```python
from build123d import *

# Parameters (mm, degrees)
SKETCH1_R          = 2.54
EXTRUDE1_DEPTH     = 20.574
SKETCH2_R          = 19.05
EXTRUDE2_DEPTH     = 1.524
SKETCH3_R          = 3.175
EXTRUDE3_DEPTH     = 20.574
EXTRUDE4_START     = -36.068
EXTRUDE4_DEPTH     = 36.068
FILLET1_R          = 2.54
EXTRUDE5_START     = 14.986
SKETCH5_R          = 3.175
EXTRUDE5_DEPTH     = 14.986
SKETCH6_R          = 1.07823
EXTRUDE6_DEPTH     = 3.81
SKETCH9_W          = 27.159483829
SKETCH9_H          = 18.094101739
CUT_EXTRUDE1_DEPTH = 56.642


with BuildPart() as part:
    # Sketch1 → Extrude1 (new, symmetric)
    with BuildSketch(Plane.XY):
        with BuildLine():
            Line((-23.5712, 28.575), (23.5712, 28.575))
            ThreePointArc((23.5712, 28.575), (27.109420912, 27.109420912), (28.575, 23.5712))
            Line((28.575, 23.5712), (28.575, -23.5712))
            ThreePointArc((28.575, -23.5712), (27.109420912, -27.109420912), (23.5712, -28.575))
            Line((23.5712, -28.575), (-23.5712, -28.575))
            ThreePointArc((-23.5712, -28.575), (-27.109420912, -27.109420912), (-28.575, -23.5712))
            Line((-28.575, -23.5712), (-28.575, 23.5712))
            ThreePointArc((-28.575, 23.5712), (-27.109420912, 27.109420912), (-23.5712, 28.575))
        make_face()
        with Locations((-23.5712, 23.5712)):
            Circle(SKETCH1_R, mode=Mode.SUBTRACT)
        with Locations((23.5712, 23.5712)):
            Circle(SKETCH1_R, mode=Mode.SUBTRACT)
        with Locations((23.5712, -23.5712)):
            Circle(SKETCH1_R, mode=Mode.SUBTRACT)
        with Locations((-23.5712, -23.5712)):
            Circle(SKETCH1_R, mode=Mode.SUBTRACT)
    extrude(amount=EXTRUDE1_DEPTH, both=True)

    # Sketch2 → Extrude2 (add)
    with BuildSketch(Plane.XY.offset(20.574)):
        with Locations(Location((0, 0, 0), (0, 0, 180))):
            Circle(SKETCH2_R)
    extrude(amount=EXTRUDE2_DEPTH)

    # Sketch3 → Extrude3 (add)
    with BuildSketch(Plane.XY.offset(20.574)):
        Circle(SKETCH3_R)
    extrude(amount=EXTRUDE3_DEPTH)

    # Sketch4 → Extrude4 (cut)
    with BuildSketch(Plane(origin=(0, 0, -20.574), x_dir=(-1, 0, 0), z_dir=(0, 0, -1)).offset(EXTRUDE4_START)):
        with BuildLine():
            Line((-23.5712, 18.5674), (-28.575, 18.5674))
            Line((-28.575, 18.5674), (-28.575, 23.5712))
            ThreePointArc((-28.575, 23.5712), (-27.109420912, 27.109420912), (-23.5712, 28.575))
            Line((-23.5712, 28.575), (-18.5674, 28.575))
            Line((-18.5674, 28.575), (-18.5674, 23.5712))
            ThreePointArc((-18.5674, 23.5712), (-20.032979088, 20.032979088), (-23.5712, 18.5674))
        make_face()
        with BuildLine():
            Line((23.5712, 18.5674), (28.575, 18.5674))
            Line((28.575, 18.5674), (28.575, 23.5712))
            ThreePointArc((28.575, 23.5712), (27.109420912, 27.109420912), (23.5712, 28.575))
            Line((23.5712, 28.575), (18.5674, 28.575))
            Line((18.5674, 28.575), (18.5674, 23.5712))
            ThreePointArc((18.5674, 23.5712), (20.032979088, 20.032979088), (23.5712, 18.5674))
        make_face()
        with BuildLine():
            Line((23.5712, -18.5674), (28.575, -18.5674))
            Line((28.575, -18.5674), (28.575, -23.5712))
            ThreePointArc((28.575, -23.5712), (27.109420912, -27.109420912), (23.5712, -28.575))
            Line((23.5712, -28.575), (18.5674, -28.575))
            Line((18.5674, -28.575), (18.5674, -23.5712))
            ThreePointArc((18.5674, -23.5712), (20.032979088, -20.032979088), (23.5712, -18.5674))
        make_face()
        with BuildLine():
            Line((-18.5674, -23.5712), (-18.5674, -28.575))
            Line((-18.5674, -28.575), (-23.5712, -28.575))
            ThreePointArc((-23.5712, -28.575), (-27.109420912, -27.109420912), (-28.575, -23.5712))
            Line((-28.575, -23.5712), (-28.575, -18.5674))
            Line((-28.575, -18.5674), (-23.5712, -18.5674))
            ThreePointArc((-23.5712, -18.5674), (-20.032979088, -20.032979088), (-18.5674, -23.5712))
        make_face()
    extrude(amount=EXTRUDE4_DEPTH, mode=Mode.SUBTRACT)

    # Fillet1
    fillet1_edges = [part.edges().sort_by_distance(p)[0] for p in [
        (28.575, -18.5674, -2.54),
        (18.5674, -28.575, -2.54),
        (18.5674, 28.575, -2.54),
        (28.575, 18.5674, -2.54),
        (-28.575, 18.5674, -2.54),
        (-18.5674, 28.575, -2.54),
        (-18.5674, -28.575, -2.54),
        (-28.575, -18.5674, -2.54),
    ]]
    fillet(fillet1_edges, radius=FILLET1_R)

    # Sketch5 → Extrude5 (add)
    with BuildSketch(Plane(origin=(0, 0, -20.574), x_dir=(-1, 0, 0), z_dir=(0, 0, -1)).offset(EXTRUDE5_START)):
        with Locations(Location((0, 0, 0), (0, 0, 180))):
            Circle(SKETCH5_R)
    extrude(amount=-EXTRUDE5_DEPTH)

    # Sketch6 → Extrude6 (cut)
    with BuildSketch(Plane(origin=(0, 0, -20.574), x_dir=(-1, 0, 0), z_dir=(0, 0, -1))):
        with Locations((-23.0124, 0)):
            Circle(SKETCH6_R)
        with Locations((23.0124, 0)):
            Circle(SKETCH6_R)
    extrude(amount=-EXTRUDE6_DEPTH, mode=Mode.SUBTRACT)

    # Sketch9 → Cut-Extrude1 (cut)
    with BuildSketch(Plane.XZ.offset(28.575)):
        with Locations((-0.774509995, -29.62105087)):
            Rectangle(SKETCH9_W, SKETCH9_H)
    extrude(amount=-CUT_EXTRUDE1_DEPTH, mode=Mode.SUBTRACT)


solid = part.part
```
Can you work these out from the model? Positions are in its coordinate system, mm. A direction names the side the tool comes from. Coordinates: 2 decimals unless noted, no trailing zeros. Loops run counter-clockwise (first coordinate to the right, second up) from the corner with the lowest first, then second, coordinate; pieces in that order, holes last. Notation, with made-up numbers: (58, 11.25) -> (103, 11.25) arc R29 ccw to (103, 34.25) -> close; hole circle Ø1 at (1, 69). An arc over 180 degrees is marked (long way). Put each result on its own line as item: value. Start each with the question number.
Q1. I'm going to push flat-ended pins straight in: P1, Ø0.6, axis at x = 23, y = 0, coming from the -Z side; P2, Ø8, axis at x = -23.57, y = 23.57, coming from the +Z side; P3, Ø4, axis at x = 23.57, y = 23.57, coming from the -Z side; P4, Ø1.2, axis at y = 25.5, z = -11, coming from the -X side. Where does each tip first touch, or does it pass through?
Q2. For faces 1 (the face through (-0.69, -3.1, 31.49)), 2 (the face through (18.567, -25, -2)), 3 (the face through (25, 18.567, -2)), 4 (the face through (-19.994, -20.072, -2.288)), 5 (the face through (-19.994, 20.072, -2.288)), which set-ups out of +Z, -Z, +X, -X, +Y, -Y let a thin tool reach every point of the face, with its end or its side?
Q3. I want a section at A-A (y = 0). Write out the boundary of the cut face in (x, z) (3 decimals).
Q4. Thinking about a two-plate mould opening in Y: for faces 6 (the face through (0, -28.575, 0)), 7 (the face through (-25.6, -25.1, 18)), 8 (the face through (-27.15, 27.07, 18.07)), which applies, pulls with the +Y half, pulls with the -Y half, needs draft (parallel to the pull), parting line crosses it, or undercut?
Q5. If I drill on line 1 (Z direction, x = -7.5, y = -3); line 2 (Z direction, x = 19, y = 14.5); line 3 (X direction, y = 26, z = -5.5), over which ranges is the centre line in solid material (lowest first)? Write a range as [from, to].
Q6. I want a section at D-D (y = 22.5). Write out the boundary of the cut face in (x, z) (3 decimals).
Q7. I want a section at C-C (x = 0). Write out the boundary of the cut face in (y, z) (3 decimals), plus the area to 3 significant figures.
Q8. I want a section at B-B (z = -11). Write out the boundary of the cut face in (x, y) (3 decimals).
Taken from the geometry:
1. P1: stops at z = -16.76
1. P2: stops at z = 20.57
1. P3: passes through
1. P4: stops at x = -18.57
2. face 1: +Z
2. face 2: -Z, +X, -Y
2. face 3: -Z, +X, +Y
2. face 4: -Z, -X, -Y
2. face 5: -Z, -X, +Y
3. outline: (-28.575, -20.574) -> (-24.091, -20.574) -> (-24.091, -16.764) -> (-21.934, -16.764) -> (-21.934, -20.574) -> (21.934, -20.574) -> (21.934, -16.764) -> (24.091, -16.764) -> (24.091, -20.574) -> (28.575, -20.574) -> (28.575, 20.574) -> (19.05, 20.574) -> (19.05, 22.098) -> (3.175, 22.098) -> (3.175, 41.148) -> (-3.175, 41.148) -> (-3.175, 22.098) -> (-19.05, 22.098) -> (-19.05, 20.574) -> (-28.575, 20.574) -> close
4. face 6: pulls with the -Y half
4. face 7: undercut
4. face 8: pulls with the +Y half
5. line 1: z = [-20.57, 22.1]
5. line 2: z = [-20.57, 20.57]
5. line 3: x = [-18.57, 18.57]
6. outline: (-28.575, 15.494) -> (-25.874, 15.494) -> (-25.874, 20.574) -> (-28.575, 20.574) -> close; (-21.268, 15.494) -> (-18.683, 15.494) -> (-18.683, -20.574) -> (18.683, -20.574) -> (18.683, 15.494) -> (21.268, 15.494) -> (21.268, 20.574) -> (-21.268, 20.574) -> close; (25.874, 15.494) -> (28.575, 15.494) -> (28.575, 20.574) -> (25.874, 20.574) -> close
7. outline: (-28.575, -20.574) -> (28.575, -20.574) -> (28.575, 20.574) -> (19.05, 20.574) -> (19.05, 22.098) -> (3.175, 22.098) -> (3.175, 41.148) -> (-3.175, 41.148) -> (-3.175, 22.098) -> (-19.05, 22.098) -> (-19.05, 20.574) -> (-28.575, 20.574) -> close
7. area: 2,530 mm2
8. outline: (-28.575, -16.027) arc R2.54 ccw to (-26.035, -18.567) -> (-23.571, -18.567) arc R5.004 cw to (-18.567, -23.571) -> (-18.567, -26.035) arc R2.54 ccw to (-16.027, -28.575) -> (16.027, -28.575) arc R2.54 ccw to (18.567, -26.035) -> (18.567, -23.571) arc R5.004 cw to (23.571, -18.567) -> (26.035, -18.567) arc R2.54 ccw to (28.575, -16.027) -> (28.575, 16.027) arc R2.54 ccw to (26.035, 18.567) -> (23.571, 18.567) arc R5.004 cw to (18.567, 23.571) -> (18.567, 26.035) arc R2.54 ccw to (16.027, 28.575) -> (-16.027, 28.575) arc R2.54 ccw to (-18.567, 26.035) -> (-18.567, 23.571) arc R5.004 cw to (-23.571, 18.567) -> (-26.035, 18.567) arc R2.54 ccw to (-28.575, 16.027) -> close
